Check sheet for the drawn part. Datum: minimum x, y, z corner. Units: mm. Coordinates: 2 decimals unless noted, no trailing zeros. Write each loop counter-clockwise with the first axis right and the second up, starting at its lowest first coordinate (ties: lowest second). Pieces come first, ordered by that corner, then holes. Notation, with made-up numbers: M 89.5,15 L 93.5,15 A25 ccw 93.5,27 Z; hole C 79,79.5 d2. An arc over 180 degrees is marked long. Answer as CSV lines item,"result". Start each with the question number.
Q1. Sectioned sample at C-C, the plane x = 39. Record the cut outline in (y, z).
Q2. Thickness scan on line 1 along Z through (x, y) = (14, 3.6) (1 decimal); line 2 along Z through (x, y) = (60, 3.4); line 3 along Z through (x, y) = (73, 0.4). Record the ranges inside material, lowest first. Write a range as from..to.
Q3. Sectioned sample at D-D, the plane z = 10.5. Record the cut outline in (x, y) (3 decimals).
Q4. Depth check by flat-ended pin: pin 1 Ø1.1 at (y, z) = (2.5, 46.5) entering from +X; pin 2 Ø1.5 at (y, z) = (2, 72.5) entering from +X; pin 3 Ø1.1 at (x, y) = (39, 1.5) entering from +Z. Enter the tip coordinate at first touch or a pass-through.
Q5. Sectioned sample at B-B, the plane y = 1.2. Record the cut outline in (x, z), then the cut area to 3 significant figures.
Q6. Sectioned sample at A-A, the plane z = 70.5. Record the cut outline in (x, y) (3 decimals).
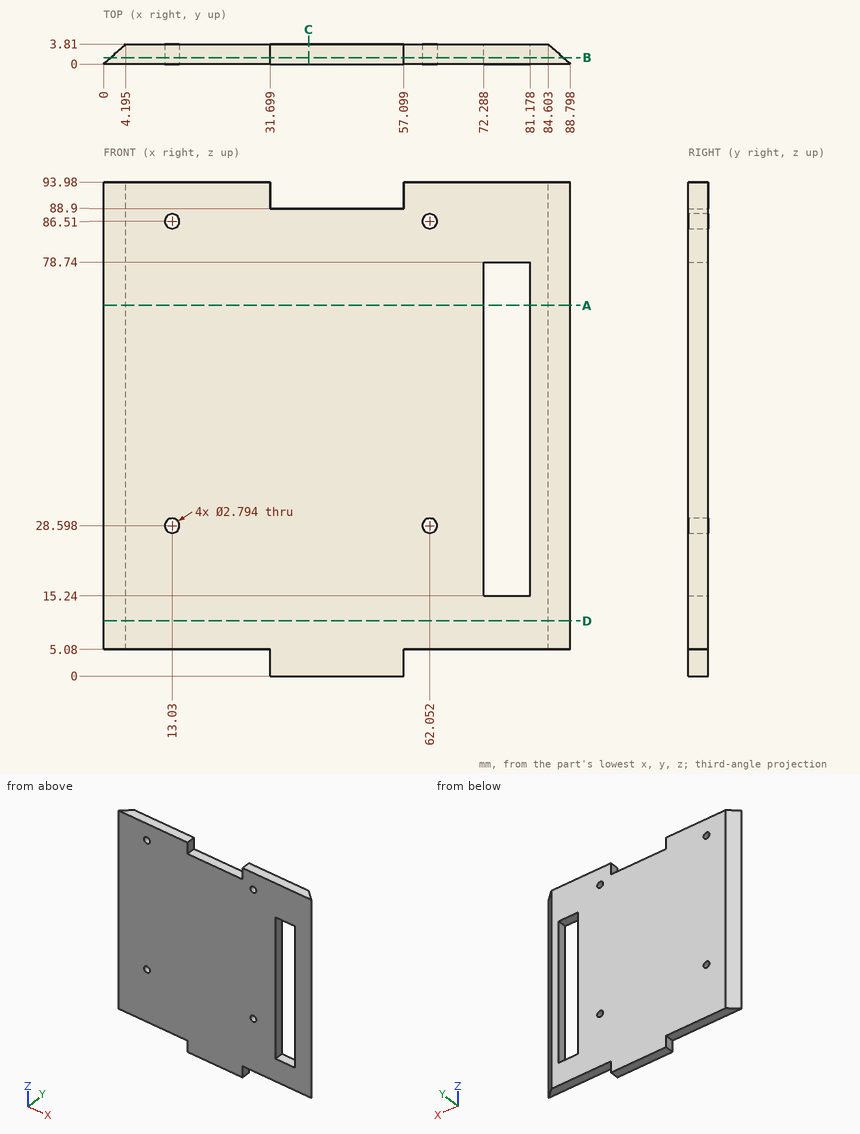
Output:
1,outline,"M 0,0 L 3.81,0 L 3.81,88.9 L 0,88.9 Z"
2,line 1,"z = 5.1..27.6, 29.6..85.5, 87.5..94"
2,line 2,"z = 5.08..93.98"
2,line 3,"z = 5.08..15.24, 78.74..93.98"
3,outline,"M 0,0 L 88.798,0 L 84.603,3.81 L 4.195,3.81 Z"
4,pin 1,"stops at x = 86.65"
4,pin 2,"stops at x = 87.42"
4,pin 3,"stops at z = 88.9"
5,outline,"M 1.32,5.08 L 31.7,5.08 L 31.7,0 L 57.1,0 L 57.1,5.08 L 87.48,5.08 L 87.48,93.98 L 57.1,93.98 L 57.1,88.9 L 31.7,88.9 L 31.7,93.98 L 1.32,93.98 Z; hole C 13.03,28.6 d2.79; hole C 13.03,86.51 d2.79; hole C 62.05,28.6 d2.79; hole C 62.05,86.51 d2.79; hole M 72.29,15.24 L 81.18,15.24 L 81.18,78.74 L 72.29,78.74 Z"
5,area,"7,070 mm^2"
6,outline,"M 0,0 L 72.288,0 L 72.288,3.81 L 4.195,3.81 Z; M 81.178,0 L 88.798,0 L 84.603,3.81 L 81.178,3.81 Z"
